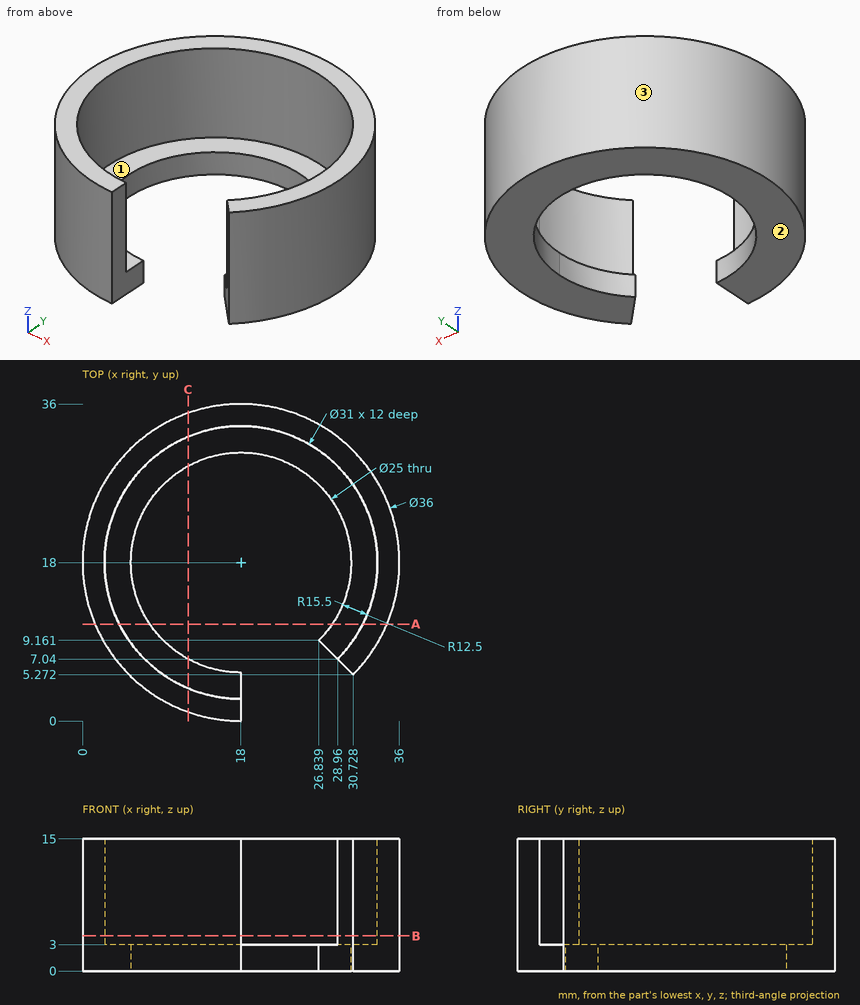
Geometry: see drawing. Coordinates: mm, zero at the bounding-box minimum. Coordinates: 2 decimals unless noted, no trailing zeros. Order: outer loops, then holes, each group sorted by start corner. A loop starts at its lowest first (then second) coordinate and runs counter-clockwise, first axis right, second up. Notation, with made-up numbers: M 19.25,-33 L 49.25,-33 A33 ccw 49.25,4 Z; hole C -18,-9 d9. An arc over 180 degrees is marked long. Answer in a Markdown table with one row per item. Add a question column.
Q1. Line query: L1, parallel to Y at x = 15, z = 2.5 (1 decimal); L2, parallel to X at y = 32, z = 4 (1 decimal); L3, parallel to Y at x = 8, z = 9.75. Output: solid intervals per line, ascending.
Q2. Section query B-B on z = 4. Return the cut outline in (x, y), and give its area (3 significant figures).
Q3. Section query C-C on x = 12. Return the cut outline in (y, z).
Q4. Contact query for flat-ended pins moving along their axis: P1, Ø8, axis at x = 30, z = 5.5, coming from the +Y side; P2, Ø4, axis at x = 11.5, z = 9, coming from the -Y side; P3, Ø1, axis at x = 28, z = 10, coming from the -Y side; P4, Ø18.5, axis at x = 18, y = 18, coming from the +Z side. Output: stop coordinate, or through.
Q5. Mould query, pull axis X, two halves, no side actions, for the marked faces 1, 2 and 3. Classes: released by +X, released by -X, zero draft, split by the parting line, or undercut.
Q6. Section query A-A on y = 11. Return the cut outline in (x, z).
Completed:
| question | item | result |
|---|---|---|
| 1 | L1 | y = 0.3 to 5.9, 30.1 to 35.7 |
| 1 | L2 | x = 6.7 to 11.3, 24.7 to 29.3 |
| 1 | L3 | y = 3.03 to 6.16, 29.84 to 32.97 |
| 2 | outline | M 18,0 L 18,2.5 A15.5 cw long 28.96,7.04 L 30.73,5.27 A18 ccw long Z |
| 2 | area | 230 mm2 |
| 3 | outline | M 1.03,0 L 7.03,0 L 7.03,3 L 3.71,3 L 3.71,15 L 1.03,15 Z; M 28.97,0 L 34.97,0 L 34.97,15 L 32.29,15 L 32.29,3 L 28.97,3 Z |
| 4 | P1 | stops at y = 34.12 |
| 4 | P2 | stops at y = 0.57 |
| 4 | P3 | stops at y = 29.4 |
| 4 | P4 | passes through |
| 5 | face 1 | undercut |
| 5 | face 2 | zero draft |
| 5 | face 3 | split by the parting line |
| 6 | outline | M 1.42,0 L 7.64,0 L 7.64,3 L 4.17,3 L 4.17,15 L 1.42,15 Z; M 28.36,0 L 34.58,0 L 34.58,15 L 31.83,15 L 31.83,3 L 28.36,3 Z |
